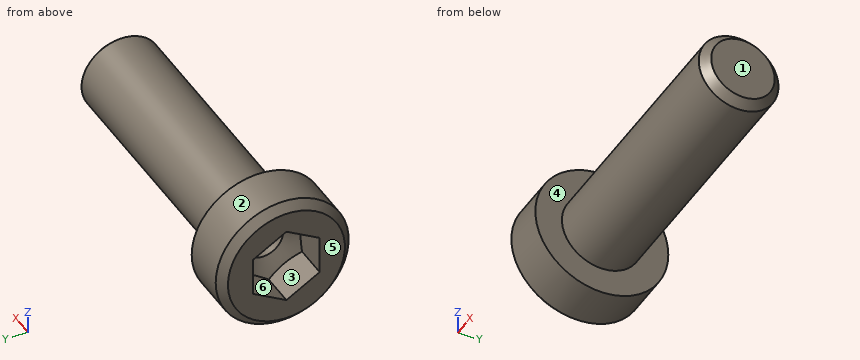
Autodesk Inventor part; units mm, degrees
ref_plane "Work Plane1" through (10, 0, 0) normal (0, 0.5, 0.866) x (1, 0, 0)
ref_plane "YZ Plane" through (0, 0, 0) normal (1, 0, 0) x (0, 1, 0)
ref_plane "XZ Plane" through (0, 0, 0) normal (0, 1, 0) x (-1, 0, 0)
sketch "Skizze1" plane through (0, 0, 0) normal (0, 0, 1) x (1, 0, 0)
  line L0 (1.866, 0) -> (20, 0)
  line L1 (20, 0) -> (20, 3)
  line L2 (20, 3) -> (0, 3)
  line L3 (0, 3) -> (0, 5)
  line L4 (0, 5) -> (-4, 5)
  line L5 (-4, 5) -> (-4, 2.8868)
  line L6 (-4, 2.8868) -> (-1.5, 2.8868)
  line L7 (-1.5, 2.8868) -> (-0.6994, 1.5)
  line L8 (-8.8, 0) -> (24.8, 0)
  line L9 (0, -1) -> (0, 6)
  line L10 (-0.6994, 1.5) -> (1, 1.5)
  line L11 (1, 1.5) -> (1.866, 0)
  line L12 (-4, 2.8868) -> (-4, 0) construction
  line L13 (-4, 4.4) -> (-3.4, 5)
  dimension "d0" = 4
  dimension "d1" = 2.5
  dimension "d2" = 60
  dimension "d3" = 6
  dimension "d4" = 5.7735
  dimension "d5" = 10
  dimension "d15" = 5
  dimension "d16" = 3
  dimension "d17" = 20
  dimension "d32" = 45
  dimension "d33" = 0.6
revolve "Körper" add sketch "Skizze1" angle 360 about axis through (1.866, 0, 0) along (1, 0, 0) contours L11 L10 L9 L2 L1 L0 | L10 L7 L6 L5 L13 L4 L3 L9 | L13 L5 L4
revolve "Fase2" cut sketch "Skizze1" angle 360 about axis through (-10, 0, 0) along (1, 0, 0) contours L13 L5 L4
sketch "Skizze2" plane through (-4, 0, 0) normal (-1, 0, 0) x (0, 0, 1)
  circle A0 centre (0, 0) radius 2.8868
  line L0 (0, -7) -> (0, 7)
  line L1 (-7, 0) -> (7, 0)
  line L2 (2.8868, 0) -> (1.4434, -2.5)
  line L3 (1.4434, -2.5) -> (-1.4434, -2.5)
  line L4 (-1.4434, -2.5) -> (-2.8868, 0)
  line L5 (-2.8868, 0) -> (-1.4434, 2.5)
  line L6 (-1.4434, 2.5) -> (1.4434, 2.5)
  line L7 (1.4434, 2.5) -> (2.8868, 0)
extrude "Loch" add sketch "Skizze2" against normal up to next contours L7 A0 | A0 L2 | L6 L0 A0 | A0 L0 L3 | L0 L6 A0 | A0 L3 L0 | L4 A0 | A0 L5
thread "Gewinde"
chamfer "Fase1" distance 0.6135 distance2 0.6135 1 edges at (20, -3, 0) measured on face at (20, 1.0659, 1.0214)
ref_plane "Work Plane1" through (10, 0, 0) normal (0, 0.5, 0.866) x (1, 0, 0)
equation "\"d0\" = KOH"
equation "\"d1\" = INTI"
equation "\"d3\" = GD"
equation "\"d4\" = 1.1547 * SW"
equation "\"d5\" = KOD"
equation "\"d15\" = INFT"
equation "\"d16\" = SDT"
equation "\"d17\" = NLG"
equation "\"d33\" = Cham"
equation "\"d7\" = GEL"
equation "\"d9\" = -0.5 * SPD + 0.5 * GD"
equation "\"d12\" = GUL"
equation "\"GD\" = NND"
equation "\"NLG\" = 20"
equation "\"GEL\" = 14.5"
equation "\"KOD\" = 10"
equation "\"KOH\" = 4"
equation "\"GUL\" = 0.61345 * PTC"
equation "\"SW\" = 5"
equation "\"INTI\" = 2.5"
equation "\"SPD\" = NND - 1.2269 * PTC"
equation "\"SDT\" = 3"
equation "\"INFT\" = 5"
equation "\"Cham\" = 0.6"
equation "\"TOA\" = 30deg"
equation "\"GD1\" = THREADDIA - 1.2269 * PTC"
equation "\"THREADDIA\" = 6"
equation "\"BDM\" = NND"
equation "\"FAWI\" = 45deg"
equation "\"RR\" = 0.1 * NND"
equation "\"PTC\" = 1"
equation "\"NND\" = 6"
equation "\"FAWI1\" = 45deg"
equation "\"GAL\" = 0.61345 * PTC"
equation "\"E0\" = 1.155 * SW"
properties part number "DIN 6912 - M6 x 20" material "Stahl, weich"
Here's how the part is built. I have some questions about the finished solid (model axes, mm). Face numbers are marked on the shaded views. A direction names the side the tool comes from. Round coordinates to 2 decimals unless told otherwise and drop trailing zeros. Order: outer loops, then holes, each group sorted by start corner. A loop starts at its lowest first (then second) coordinate and runs counter-clockwise, first axis right, second up. Notation, with made-up numbers: (-39, 0.25) -> (0, 0.25) arc R25 ccw to (0, 19.25) -> close; hole circle Ø3 at (29, -39.75). An arc over 180 degrees is marked (long way). Use a Markdown table: item, result. Add a question column.
(1) For the marked faces 4, 5 and 6, which set-ups out of +Z, -Z, +X, -X, +Y, -Y let a thin tool reach every point of the face, with its end or its side?
(2) I need wall thicknesses on line 1 along Z through (x, y) = (-0.05, 0); line 2 along Z through (x, y) = (0.4, 0); line 3 along X through (y, z) = (-4.25, -0.5). Which ranges of each line are inside material? Lowest first, please.
(3) For pin 1 Ø3 at (x, z) = (-3, -0.5) entering from -Y; pin 2 Ø3 at (x, z) = (6, 3) entering from -Y; pin 3 Ø2.5 at (y, z) = (0, 0) entering from -X; pin 4 Ø2 at (y, z) = (3, -4) entering from +X, each with a flat end and sliding along its axis, tell me the tip position at first contact or that it passes through.
(4) Suppose I cut it at B-B, the plane x = 1.5. Please give me the cut outline in (y, z).
(5) Suppose I cut it at A-A, the plane x = 12.5. Please give me the cut outline in (y, z).
(6) If we mould it in two halves opening along Z, with no side actions, what happens to the marked faces 1, 2 and 3? For each: released by +Z, released by -Z, zero draft, split by the parting line, or undercut.
Verdict:
| question | item | result |
|---|---|---|
| 1 | face 4 | +X |
| 1 | face 5 | +Z, -Z, -X, +Y, -Y |
| 1 | face 6 | -X |
| 2 | line 1 | -5 to -1.5, 1.5 to 5 |
| 2 | line 2 | -3 to -1.5, 1.5 to 3 |
| 2 | line 3 | -4 to 0 |
| 3 | pin 1 | y = -5 |
| 3 | pin 2 | y = -2.6 |
| 3 | pin 3 | x = 1.14 |
| 3 | pin 4 | x = 0 |
| 4 | outline | circle Ø6 at (0, 0); hole circle Ø1.27 at (0, 0) |
| 5 | outline | circle Ø6 at (0, 0) |
| 6 | face 1 | zero draft |
| 6 | face 2 | split by the parting line |
| 6 | face 3 | undercut |
